from build123d import *

# Parameters (mm, degrees)
SKETCH_1_R      = 5.6
SKETCH_1_R_2    = 4
EXTRUDE_1_DEPTH = 6
CHAMFER_1_SIZE  = 0.3
CHAMFER_2_SIZE  = 0.4


with BuildPart() as part:
    # Эскиз1 → Бобышка-Вытянуть1 (new body)
    with BuildSketch(Plane(origin=(0, 0, 0), x_dir=(1, 0, 0), z_dir=(0, 1, 0))):
        with Locations(Location((0, 0, 0), (0, 0, 270))):
            Circle(SKETCH_1_R)
        with Locations(Location((0, 0, 0), (0, 0, 270))):
            Circle(SKETCH_1_R_2, mode=Mode.SUBTRACT)
    extrude(amount=EXTRUDE_1_DEPTH)

    # Фаска1
    chamfer_1_edges = [part.edges().sort_by_distance(p)[0] for p in [
        (0, 0, -4),
        (0, 6, -4),
    ]]
    chamfer(chamfer_1_edges, length=CHAMFER_1_SIZE)

    # Фаска2
    chamfer_2_edges = [part.edges().sort_by_distance(p)[0] for p in [
        (0, 0, -5.6),
        (0, 6, -5.6),
    ]]
    chamfer(chamfer_2_edges, length=CHAMFER_2_SIZE)


solid = part.part
Design review of the part built by this model. Coordinates are the model's own, in mm. Round coordinates to 2 decimals unless told otherwise and drop trailing zeros. Write each loop counter-clockwise with the first axis right and the second up, starting at its lowest first coordinate (ties: lowest second). Pieces come first, ordered by that corner, then holes. Notation, with made-up numbers: (-6.75, 72) -> (33.25, 72) arc R23 ccw to (33.25, 102) -> close; hole circle Ø5 at (-7, -4). An arc over 180 degrees is marked (long way). One line per item, written item: value. Start each with the question number.
Q1. Add section C-C (y = 3.1). Give the boundary of the cut face in (x, z).
Q2. Add section A-A (z = 0). Give the boundary of the cut face in (x, y), then the cut area to 3 significant figures.
Q3. Insertion check: P1, Ø1, axis at x = 4, y = 4.5, coming from the -Z side. The pin has a flat end and moves straight along its axis. Give the tip position at first contact, or say it passes through.
Q4. Add section B-B (x = 0). Give the boundary of the cut face in (y, z).
Q5. To check wall thickness, follow probe 1 along X at (y, z) = (3.75, 0); probe 2 along X at (y, z) = (1.45, -3); probe 3 along Z at (x, y) = (-3.5, 3.25). State the ranges of each line that lie inside material, in increasing order.
Q6. The part is to be moulded in two halves that separate along Z. For faces 1 (the face through (4, 6, -2)), 2 (the face through (0.246, 2.964, -5.595)), 3 (the face through (-3.905, 2.962, -0.867)), say which applies: pulls with the +Z half, pulls with the -Z half, needs draft (parallel to the pull), parting line crosses it, or undercut.
Response:
1. outline: circle Ø11.2 at (0, 0); hole circle Ø8 at (0, 0)
2. outline: (-5.6, 0.4) -> (-5.2, 0) -> (-4.3, 0) -> (-4, 0.3) -> (-4, 5.7) -> (-4.3, 6) -> (-5.2, 6) -> (-5.6, 5.6) -> close; (4, 0.3) -> (4.3, 0) -> (5.2, 0) -> (5.6, 0.4) -> (5.6, 5.6) -> (5.2, 6) -> (4.3, 6) -> (4, 5.7) -> close
2. area: 18.7 mm^2
3. P1: stops at z = -4.37
4. outline: (0, -5.2) -> (0.4, -5.6) -> (5.6, -5.6) -> (6, -5.2) -> (6, -4.3) -> (5.7, -4) -> (0.3, -4) -> (0, -4.3) -> close; (0, 4.3) -> (0.3, 4) -> (5.7, 4) -> (6, 4.3) -> (6, 5.2) -> (5.6, 5.6) -> (0.4, 5.6) -> (0, 5.2) -> close
5. probe 1: x = -5.6 to -4, 4 to 5.6
5. probe 2: x = -4.73 to -2.65, 2.65 to 4.73
5. probe 3: z = -4.37 to -1.94, 1.94 to 4.37
6. face 1: needs draft
6. face 2: parting line crosses it
6. face 3: undercut
